Could you check a few things on this model? Use its own coordinates, in mm. A direction names the side the tool comes from. Round coordinates to 2 decimals unless told otherwise and drop trailing zeros. Write each loop counter-clockwise with the first axis right and the second up, starting at its lowest first coordinate (ties: lowest second). Pieces come first, ordered by that corner, then holes. Notation, with made-up numbers: (78.5, 53) - (93.5, 53) arc R20 ccw to (93.5, 91) - close; hole circle Ø6 at (85.25, 34). An arc over 180 degrees is marked (long way). Put each result on its own line as item: value.
from build123d import *

# Parameters (mm, degrees)
SKETCH1_R           = 8
BOSS_EXTRUDE2_DEPTH = 6
SKETCH5_R           = 12.5
BOSS_EXTRUDE3_DEPTH = 2
SKETCH6_R           = 12.5
BOSS_EXTRUDE4_DEPTH = 2
BOSS_EXTRUDE4_TAPER = 80


with BuildPart() as part:
    # Sketch1 → Boss-Extrude2 (new body)
    with BuildSketch(Plane.XY):
        Circle(SKETCH1_R)
    extrude(amount=-BOSS_EXTRUDE2_DEPTH)

    # Sketch5 → Boss-Extrude3 (add)
    with BuildSketch(Plane.XY):
        Circle(SKETCH5_R)
    extrude(amount=BOSS_EXTRUDE3_DEPTH)

    # Sketch6 → Boss-Extrude4 (add)
    with BuildSketch(Plane.XY.offset(2)):
        Circle(SKETCH6_R)
    extrude(amount=BOSS_EXTRUDE4_DEPTH, taper=BOSS_EXTRUDE4_TAPER)


solid = part.part
(1) For faces 1 (the face through (0, 0, -6)), 2 (the face through (-1.73, -7.81, -2.96)), which set-ups out of +Z, -Z, +X, -X, +Y, -Y let a thin tool reach every point of the face, with its end or its side?
Values found:
face 1: -Z, +X, -X, +Y, -Y
face 2: -Z
(2) Imagine slicing it at C-C, the plane z = -1.25. List the corners of the cut face in (x, y) for me, then the cut area to 3 significant figures.
Values found:
outline: circle Ø16 at (0, 0)
area: 201 mm^2
(3) Imagine slicing it at A-A, the plane y = 0. List the corners of the cut face in (x, z) for me.
Values found:
outline: (-12.5, 0) - (-8, 0) - (-8, -6) - (8, -6) - (8, 0) - (12.5, 0) - (12.5, 2) - (1.16, 4) - (-1.16, 4) - (-12.5, 2) - close
(4) Please list where these lines run through material, in increasing order: probe 1 along Z at (x, y) = (1.5, 8); probe 2 along Z at (x, y) = (3.75, 1.25); probe 3 along Y at (x, z) = (-8.25, 1). Write a range as from..to.
Values found:
probe 1: z = 0..2.77
probe 2: z = -6..3.51
probe 3: y = -9.39..9.39
(5) Imagine slicing it at D-D, the plane z = 3. List the corners of the cut face in (x, y) for me.
Values found:
outline: circle Ø13.66 at (0, 0)
(6) I'm going to push flat-ended pins straight in: pin 1 (2 mm diameter, centred on x = 0, z = -2.5, fed in from -Y); pin 2 (1.5 mm diameter, centred on y = 0.5, z = -0.5, fed in from +X); pin 3 (5 mm diameter, centred on x = 7.5, z = 0, fed in from -Y); pin 4 (3 mm diameter, centred on x = -2.5, y = -3, fed in from +Z). Where does each tip first touch, or does it pass through?
Values found:
pin 1: stops at y = -8
pin 2: stops at x = 12.5
pin 3: stops at y = -11.46
pin 4: stops at z = 3.78
